Source: CAD feature listing. Evaluate the final solid. Frame: model axes, mm. Face numbers are marked on the shaded views. Coordinates: 2 decimals unless noted, no trailing zeros. Order: outer loops, then holes, each group sorted by start corner. A loop starts at its lowest first (then second) coordinate and runs counter-clockwise, first axis right, second up.
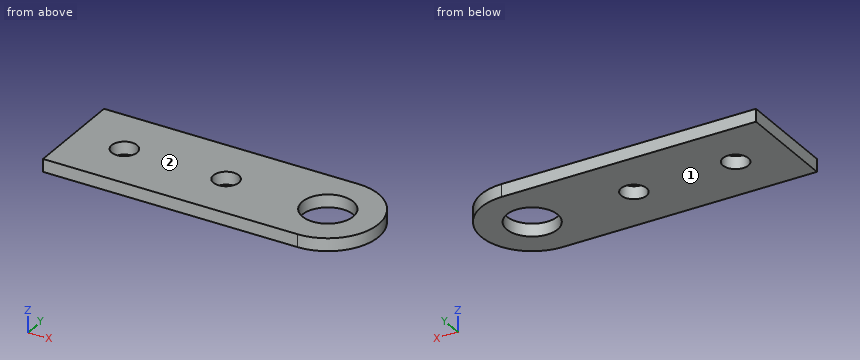
```python
from build123d import *

# Parameters (mm, degrees)
SKETCH1_R          = 6.35
SKETCH1_R_2        = 3.175
BASE_FLANGE1_DEPTH = 3.175


# Sheet-metal steps are written as plain solids
with BuildPart() as part:
    # Sketch1 → Base-Flange1 (new body)
    with BuildSketch(Plane.XY):
        with BuildLine():
            Line((0, 12.7), (-63.5, 12.7))
            Line((-63.5, 12.7), (-63.5, -12.7))
            Line((-63.5, -12.7), (0, -12.7))
            ThreePointArc((0, -12.7), (12.7, 0), (0, 12.7))
        make_face()
        Circle(SKETCH1_R, mode=Mode.SUBTRACT)
        with Locations((-50.8, 0)):
            Circle(SKETCH1_R_2, mode=Mode.SUBTRACT)
        with Locations((-25.4, 0)):
            Circle(SKETCH1_R_2, mode=Mode.SUBTRACT)
    extrude(amount=-BASE_FLANGE1_DEPTH)


solid = part.part
```
Q1. Section query D-D on x = 5. Output: boundary loops of the cut face in (y, z) (3 decimals), plus the area to 3 significant figures.
Solutions:
outline: (-11.674, -3.175) - (-3.914, -3.175) - (-3.914, 0) - (-11.674, 0) - close; (3.914, -3.175) - (11.674, -3.175) - (11.674, 0) - (3.914, 0) - close
area: 49.3 mm2
Q2. Material intervals for line 1 along X through (y, z) = (0.25, -1.65); line 2 along Y through (x, z) = (-51, -1.4); line 3 along X through (y, z) = (-1, -2.95), sorted ascending.
Solutions:
line 1: x = -63.5 to -53.97, -47.63 to -28.57, -22.23 to -6.35, 6.35 to 12.7
line 2: y = -12.7 to -3.17, 3.17 to 12.7
line 3: x = -63.5 to -53.81, -47.79 to -28.41, -22.39 to -6.27, 6.27 to 12.66
Q3. Section query B-B on x = -25.4. Output: boundary loops of the cut face in (y, z) (3 decimals), plus the area to 3 significant figures.
Solutions:
outline: (-12.7, -3.175) - (-3.175, -3.175) - (-3.175, 0) - (-12.7, 0) - close; (3.175, -3.175) - (12.7, -3.175) - (12.7, 0) - (3.175, 0) - close
area: 60.5 mm2
Q4. Pin query (flat end, axial travel): P1, Ø1, axis at y = -1.5, z = -0.5, coming from the +X side. Return the tip coordinate at first contact, or that it passes through.
Solutions:
P1: stops at x = 12.66
Q5. Pull-direction query (Z, two-part tool) for the marked faces 1 and 2; classes: pulls with the +Z half, pulls with the -Z half, needs draft (parallel to the pull), parting line crosses it, or undercut.
Solutions:
face 1: pulls with the -Z half
face 2: pulls with the +Z half
Q6. Section query C-C on z = -0.5. Output: boundary loops of the cut face in (x, y) (3 decimals).
Solutions:
outline: (-63.5, -12.7) - (0, -12.7) arc R12.7 ccw to (0, 12.7) - (-63.5, 12.7) - close; hole circle Ø6.35 at (-50.8, 0); hole circle Ø6.35 at (-25.4, 0); hole circle Ø12.7 at (0, 0)
Q7. Section query A-A on y = 0. Output: boundary loops of the cut face in (x, z) (3 decimals), plus the area to 3 significant figures.
Solutions:
outline: (-63.5, -3.175) - (-53.975, -3.175) - (-53.975, 0) - (-63.5, 0) - close; (-47.625, -3.175) - (-28.575, -3.175) - (-28.575, 0) - (-47.625, 0) - close; (-22.225, -3.175) - (-6.35, -3.175) - (-6.35, 0) - (-22.225, 0) - close; (6.35, -3.175) - (12.7, -3.175) - (12.7, 0) - (6.35, 0) - close
area: 161 mm2
